from build123d import *

# Parameters (mm, degrees)
PAD_DEPTH       = 80
SKETCH001_W     = 13.46115
SKETCH001_H     = 25.548716
POCKET_DEPTH    = 5
POCKET001_DEPTH = 5
POCKET002_DEPTH = 2.5
POCKET003_DEPTH = 2.5


with BuildPart() as part:
    # Sketch → Pad (new body)
    with BuildSketch(Plane.XZ):
        Polygon((0, 29.595964), (-29.898989, 0), (-29.898989, -40.505043), (29.898993, -40.505043), (29.898993, 0), align=None)
    extrude(amount=PAD_DEPTH)

    # Sketch001 (on Face7 of Pad) → Pocket (cut)
    with BuildSketch(Plane.XZ.offset(80)):
        with Locations((-13.049075, -28.256087)):
            Rectangle(SKETCH001_W, SKETCH001_H)
    extrude(amount=-POCKET_DEPTH, mode=Mode.SUBTRACT)

    # Sketch002 (on Face5 of Pocket) → Pocket001 (cut)
    with BuildSketch(Plane.XZ.offset(80)):
        Polygon((0, 25.160156), (-26.375223, 0), (26.642376, 0), align=None)
    extrude(amount=-POCKET001_DEPTH, mode=Mode.SUBTRACT)

    # Sketch004 (on Face5 of Pocket001) → Pocket002 (cut)
    with BuildSketch(Plane.XZ.offset(80)):
        Polygon((23.345951, -13.298216), (18.126602, -13.298216), (18.126602, -5.881243), (22.796553, -5.881243), align=None)
        Polygon((8.786701, -18.517565), (12.907252, -18.517565), (13.181961, -25.934531), (9.061434, -25.659827), align=None)
        Polygon((18.126602, -17.693453), (18.950702, -25.110434), (23.345937, -24.561026), (23.345937, -17.144047), align=None)
    extrude(amount=-POCKET002_DEPTH, mode=Mode.SUBTRACT)

    # Sketch003 (on Face5 of Pocket001) → Pocket003 (cut)
    with BuildSketch(Plane.XZ.offset(80)):
        Polygon((7.687895, -6.155951), (7.962603, -15.221137), (13.731359, -15.221137), (13.456652, -5.881243), align=None)
    extrude(amount=-POCKET003_DEPTH, mode=Mode.SUBTRACT)


solid = part.part
Work out the finished part from the listing and answer in its coordinate system (mm). A direction names the side the tool comes from. Round coordinates to 2 decimals unless told otherwise and drop trailing zeros. Loops run counter-clockwise (first coordinate to the right, second up) from the corner with the lowest first, then second, coordinate; pieces in that order, holes last. Notation, with made-up numbers: M -29.75,9.25 L -16.75,9.25 A20 cw -16.75,26.25 Z; hole C 76.5,27 d6. An arc over 180 degrees is marked long. One line per question, with ' | ' between items. Start each with the question number.
(1) A cutting plane is placed at B-B on x = 15. Write down the section's boundary in (y, z), plus the area to 3 significant figures.
(2) A tool of negligible diameter and unlimited length cuts with its end or side. For faces 5 (the face through (-13, -78, -15.482)), 6 (the face through (0, -75, 10)), 7 (the face through (-29.899, -39, -20)), from which of +Z, -Z, +X, -X, +Y, -Y can it reach the whole face along a straight path? Write none if from no direction.
(3) Find the intervals of material crossed by line 1 (Y direction, x = -19, z = -25); line 2 (Z direction, x = -3, y = -44); line 3 (X direction, y = -29.5, z = 16), in increasing order.
(4) For a pull along X with two mould halves and no side action, classify faces 1 (the face through (0, -80, -21)), 2 (the face through (-14.74, -39.44, 15.005)), 3 (the face through (8.926, -78.768, -22.139)), 4 (the face through (18.533, -78.768, -21.35)) as released by +X, released by -X, zero draft, split by the parting line, or undercut.
(5) A cutting plane is placed at C-C on z = -23. Write down the section's boundary in (x, y).
(6) Flat-ended cylindrical pins translate along their axes: pin 1 Ø2 at (x, z) = (11.5, -22) entering from -Y; pin 2 Ø2 at (x, y) = (11, -79) entering from +Z; pin 3 Ø12 at (x, y) = (14.5, -20) entering from +Z; pin 4 Ø1.5 at (x, z) = (-22.5, -26) entering from +Y. Find the tip coordinate at first contact, or state that the pin passes through.
(7) A cutting plane is placed at D-D on x = -15. Write down the section's boundary in (y, z).
(8) A cutting plane is placed at A-A on y = -20.5. Write down the section's boundary in (x, z), plus the area to 3 significant figures.
Geometry check:
1) outline: M -80,-40.51 L 0,-40.51 L 0,14.75 L -80,14.75 L -80,10.99 L -75,10.99 L -75,0 L -80,0 Z | area: 4,370 mm²
2) face 5: -Z, -Y | face 6: -Y | face 7: +Z, -Z, -X, +Y, -Y
3) line 1: y = -75 to 0 | line 2: z = -40.51 to 26.63 | line 3: x = -13.74 to 13.74
4) face 1: zero draft | face 2: released by -X | face 3: undercut | face 4: undercut
5) outline: M -29.9,-80 L -19.78,-80 L -19.78,-75 L -6.32,-75 L -6.32,-80 L 8.96,-80 L 8.96,-77.5 L 13.07,-77.5 L 13.07,-80 L 18.72,-80 L 18.72,-77.5 L 23.35,-77.5 L 23.35,-80 L 29.9,-80 L 29.9,0 L -29.9,0 Z
6) pin 1: stops at y = -77.5 | pin 2: stops at z = 19.7 | pin 3: stops at z = 21.18 | pin 4: stops at y = 0
7) outline: M -80,-15.48 L -75,-15.48 L -75,-40.51 L 0,-40.51 L 0,14.75 L -80,14.75 L -80,10.85 L -75,10.85 L -75,0 L -80,0 Z
8) outline: M -29.9,-40.51 L 29.9,-40.51 L 29.9,0 L 0,29.6 L -29.9,0 Z | area: 3,310 mm²
